The drawing under review shows one solid part. Ordinate dimensions are in mm from its lowest x, y, z. A direction names the side the tool comes from. Give positions to 0.01 mm unless a question says otherwise; leave off trailing zeros. Loops run counter-clockwise (first coordinate to the right, second up) from the corner with the lowest first, then second, coordinate; pieces in that order, holes last. Notation, with made-up numbers: M 28.5,25.5 L 46.5,25.5 A14 ccw 46.5,35.5 Z; hole C 39,-20 d6. An arc over 180 degrees is marked long. Answer as CSV lines item,"result".
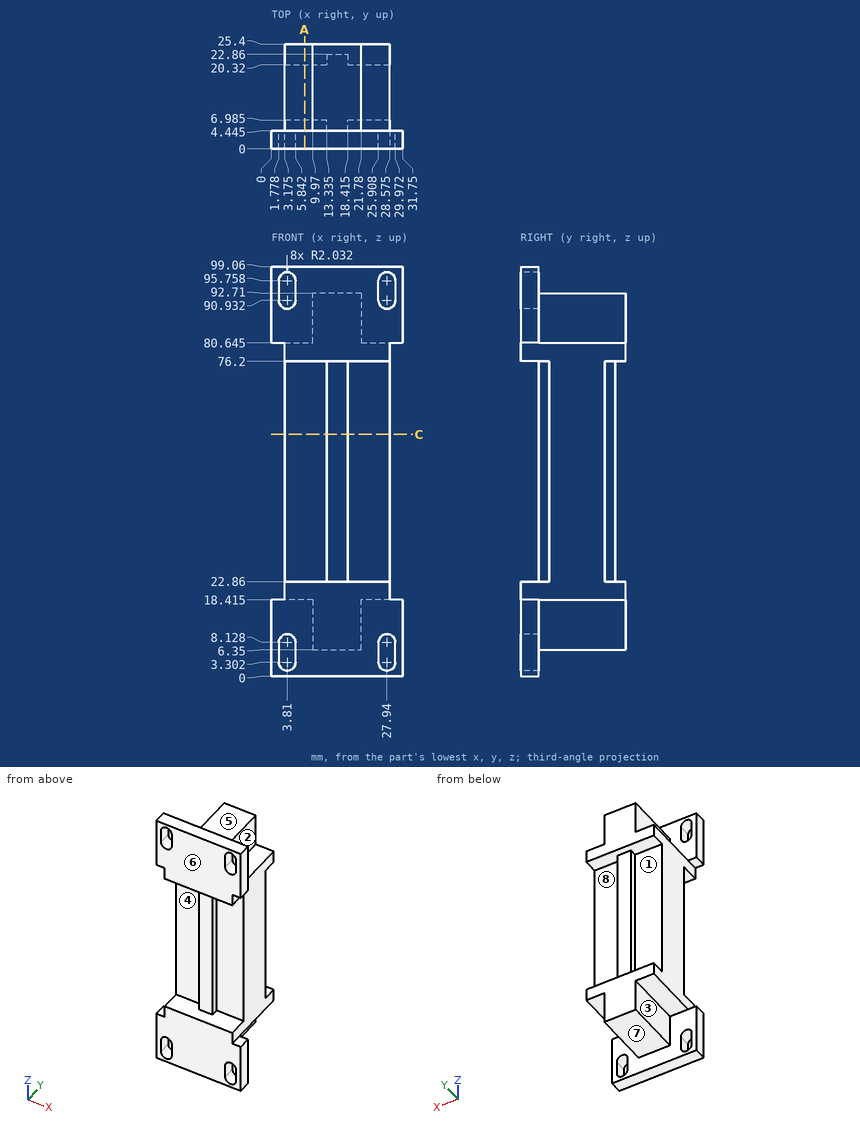
1. For P1, Ø7.5, axis at x = 24, y = 16, coming from the +Z side; P2, Ø7.5, axis at y = 17.5, z = 55.5, coming from the +X side (1 decimal); P3, Ø12, axis at y = 20, z = 38, coming from the -X side (1 decimal), all flat-tipped, find the tip position at first contact; note any pin that passes through.
Answer block:
P1,"z = 92.71"
P2,"x = 28.6"
P3,"x = 3.2"
2. To check wall thickness, follow L1, parallel to Z at x = 23.5, y = 24 (1 decimal); L2, parallel to Z at x = 12.5, y = 3; L3, parallel to X at y = 12.25, z = 54 (1 decimal). State the ranges of each line that lie inside material, in increasing order. Write a range as [from, to].
Answer block:
L1,"[18.4, 22.9], [76.2, 80.6]"
L2,"[0, 22.86], [76.2, 99.06]"
L3,"[3.2, 28.6]"
3. We need section A-A, the plane x = 8. Write out the cut boundary in (y, z) (1 decimal).
Answer block:
outline,"M 0,0 L 4.4,0 L 4.4,18.4 L 25.4,18.4 L 25.4,22.9 L 20.3,22.9 L 20.3,76.2 L 25.4,76.2 L 25.4,80.6 L 4.4,80.6 L 4.4,99.1 L 0,99.1 L 0,76.2 L 7,76.2 L 7,22.9 L 0,22.9 Z"
4. The part is to be moulded in two halves that separate along Z. For the marked faces 6, 7 and 8, say which applies: pulls with the +Z half, pulls with the -Z half, needs draft (parallel to the pull), parting line crosses it, or undercut.
Answer block:
face 6,"needs draft"
face 7,"pulls with the -Z half"
face 8,"undercut"
5. We need section C-C, the plane z = 58.5. Write out the cut boundary in (x, y) (1 decimal).
Answer block:
outline,"M 3.2,7 L 13.3,7 L 13.3,4.4 L 18.4,4.4 L 18.4,7 L 28.6,7 L 28.6,20.3 L 18.4,20.3 L 18.4,22.9 L 13.3,22.9 L 13.3,20.3 L 3.2,20.3 Z"
6. For the marked faces 1, 2, 3, 4 and 5, list the 3-axis set-ups (+Z, -Z, +X, -X, +Y, -Y) from which the entire face can be reached by the end or side of a thin tool; tool diameter is ignored.
Answer block:
face 1,"-X, +Y"
face 2,"+Z, +X, +Y"
face 3,"-Z, -X, +Y"
face 4,"-X, -Y"
face 5,"+Z, +X, -X, +Y"
